```python
from build123d import *

# Parameters (mm, degrees)
SKETCH1_W           = 69
SKETCH1_H           = 83
SKETCH1_R           = 2.25
BOSS_EXTRUDE1_DEPTH = 1.5
SKETCH2_W           = 12.7
SKETCH2_H           = 75
SKETCH2_R           = 1.5
BOSS_EXTRUDE2_DEPTH = 12.7


with BuildPart() as part:
    # Sketch1 → Boss-Extrude1 (new body)
    with BuildSketch(Plane(origin=(0, 0, 0), x_dir=(1, 0, 0), z_dir=(0, 1, 0))):
        with Locations((34.5, 41.5)):
            Rectangle(SKETCH1_W, SKETCH1_H)
        with Locations((4.5, 68.75)):
            Circle(SKETCH1_R, mode=Mode.SUBTRACT)
        with Locations((64.5, 68.75)):
            Circle(SKETCH1_R, mode=Mode.SUBTRACT)
        with Locations((64.5, 14.25)):
            Circle(SKETCH1_R, mode=Mode.SUBTRACT)
        with Locations((4.5, 14.25)):
            Circle(SKETCH1_R, mode=Mode.SUBTRACT)
    extrude(amount=BOSS_EXTRUDE1_DEPTH)

    # Sketch2 → Boss-Extrude2 (add)
    with BuildSketch(Plane(origin=(0, 1.5, 0), x_dir=(1, 0, 0), z_dir=(0, 1, 0))):
        with Locations((34.5, 40.9)):
            Rectangle(SKETCH2_W, SKETCH2_H)
        with Locations((34.5, 8.9)):
            Circle(SKETCH2_R, mode=Mode.SUBTRACT)
        with Locations((34.5, 18.9)):
            Circle(SKETCH2_R, mode=Mode.SUBTRACT)
    extrude(amount=BOSS_EXTRUDE2_DEPTH)


solid = part.part
```
Read the model definition and answer for the solid it produces. Units are mm, in the model's axes. A direction names the side the tool comes from. Round coordinates to 2 decimals unless told otherwise and drop trailing zeros. Write each loop counter-clockwise with the first axis right and the second up, starting at its lowest first coordinate (ties: lowest second). Pieces come first, ordered by that corner, then holes. Notation, with made-up numbers: M 89.25,13 L 125.25,13 A20 cw 125.25,18 Z; hole C -36.5,-25.75 d8. An arc over 180 degrees is marked long. One line per item, written item: value.
Q1. For a pull along Z with two mould halves and no side action, classify faces 5 (the flat face through (34, 0, -42)), 6 (the flat face through (34, 8, -3.4)), 7 (the cylindrical face through (62.252, 0.74, -14.349)) as +Z half, -Z half, draft (parallel to the pull), parting line (faces both ways), or undercut.
Data:
face 5: draft
face 6: +Z half
face 7: undercut
Q2. Find section C-C on x = 34.5. Write down the section's boundary in (y, z), plus the area to 3 significant figures.
Data:
outline: M 0,-83 L 1.5,-83 L 1.5,-78.4 L 14.2,-78.4 L 14.2,-20.4 L 1.5,-20.4 L 1.5,-17.4 L 14.2,-17.4 L 14.2,-10.4 L 1.5,-10.4 L 1.5,-7.4 L 14.2,-7.4 L 14.2,-3.4 L 1.5,-3.4 L 1.5,0 L 0,0 Z
area: 1,000 mm2
Q3. Straight lines are drawn through the part: line 1 (X direction, y = 0.55, z = -14.25); line 2 (Z direction, x = 34.5, y = 5.75); line 3 (Z direction, x = 4.5, y = 0.6). For each, find the intervals that lie inside material, in ascending order. Write a range as [from, to].
Data:
line 1: [0, 2.25], [6.75, 62.25], [66.75, 69]
line 2: [-78.4, -20.4], [-17.4, -10.4], [-7.4, -3.4]
line 3: [-83, -71], [-66.5, -16.5], [-12, 0]
Q4. Find section B-B on y = 6.5. Write down the section's boundary in (x, z), plus the area to 3 significant figures.
Data:
outline: M 28.15,-78.4 L 40.85,-78.4 L 40.85,-3.4 L 28.15,-3.4 Z; hole C 34.5,-18.9 d3; hole C 34.5,-8.9 d3
area: 938 mm2
Q5. Find section A-A on z = -14.25. Write down the section's boundary in (x, y), plus the area to 3 significant figures.
Data:
outline: M 0,0 L 2.25,0 L 2.25,1.5 L 0,1.5 Z; M 6.75,0 L 62.25,0 L 62.25,1.5 L 40.85,1.5 L 40.85,14.2 L 28.15,14.2 L 28.15,1.5 L 6.75,1.5 Z; M 66.75,0 L 69,0 L 69,1.5 L 66.75,1.5 Z
area: 251 mm2
Q6. Flat-ended cylindrical pins translate along their axes: pin 1 Ø1.8 at (x, z) = (34.5, -18.9) entering from +Y; pin 2 Ø8 at (x, y) = (24, 3.5) entering from -Z; pin 3 Ø4 at (y, z) = (10.5, -54.5) entering from +X. Find the tip coordinate at first contact, or state that the pin passes through.
Data:
pin 1: y = 1.5
pin 2: z = -83
pin 3: x = 40.85
Q7. Find section D-D on z = -48. Write down the section's boundary in (x, y), plus the area to 3 significant figures.
Data:
outline: M 0,0 L 69,0 L 69,1.5 L 40.85,1.5 L 40.85,14.2 L 28.15,14.2 L 28.15,1.5 L 0,1.5 Z
area: 265 mm2
Q8. Which of the six approach directions +Z, -Z, +X, -X, +Y, -Y give full straight-line access (tool end or side, diameter ignored) to faces 1 (the flat face through (28.15, 8, -40)), 2 (the flat face through (34, 8, -78.4)), 3 (the flat face through (34, 1.5, -9)), 4 (the flat face through (40.85, 8, -40))?
Data:
face 1: +Z, -Z, -X, +Y
face 2: -Z, +X, -X, +Y
face 3: +Y
face 4: +Z, -Z, +X, +Y
